Read the model definition and answer for the solid it produces. Units are mm, in the model's axes. A direction names the side the tool comes from. Round coordinates to 2 decimals unless told otherwise and drop trailing zeros. Order: outer loops, then holes, each group sorted by start corner. A loop starts at its lowest first (then second) coordinate and runs counter-clockwise, first axis right, second up. Notation, with made-up numbers: (56, 22) - (75, 22) arc R29 ccw to (75, 47) - close; hole circle Ø9 at (-6, -26.75). An arc over 180 degrees is marked (long way). Put each result on its own line as item: value. Start each with the question number.
Q1. Section B-B on x = 6 is taken. Give the vertices of the cut face in (y, z).
Q2. Section D-D on z = 76 is taken. Give the vertices of the cut face in (x, y).
Q3. For a pull along X with two mould halves and no side action, classify faces 4 (the face through (0, 92, 44)), 5 (the face through (5.916, 125.28, 64.946)), 6 (the face through (6, 75, 67)) as pulls with the +X half, pulls with the -X half, needs draft (parallel to the pull), parting line crosses it, or undercut.
Q4. Find the intervals of material crossed by line 1 along X through (y, z) = (75, 13); line 2 along Y through (x, z) = (4.5, 78); line 3 along Y through (x, z) = (8.5, 11.5), in increasing order. Write a range as from..to.
Q5. Section C-C on z = 22 is taken. Give the vertices of the cut face in (x, y).
Q6. Section A-A on y = 75 is taken. Give the vertices of the cut face in (x, z), then the cut area to 3 significant figures.
Q7. Each of these flat-tipped pins is pushed along its axis until it touches: pin 1 Ø5 at (x, y) = (6, 75) entering from -Z; pin 2 Ø6 at (x, y) = (6.5, 111) entering from +Z; pin 3 Ø5.5 at (x, y) = (6, 75) entering from +Z. Where does it stop, or does it pass through?
Q8. Which of the six approach directions +Z, -Z, +X, -X, +Y, -Y give full straight-line access (tool end or side, diameter ignored) to faces 1 (the face through (5.35, 72.07, 77.14)), 2 (the face through (5.35, 77.93, 12.32)), 3 (the face through (6, 82, 0))?
from build123d import *

# Parameters (mm, degrees)
F1_DEPTH = 12
F2_R     = 3
F3_DEPTH = 20
F4_R     = 3
F5_DEPTH = 25
F6_R     = 2
F7_DEPTH = 25
F8_W     = 60
F8_H     = 87
F9_DEPTH = 25


with BuildPart() as f1:
    # F0 (on Right) → F1 (new body)
    with BuildSketch(Plane.YZ):
        Polygon((0, 87), (0, 0), (105, 0), (145, 43.5), (105, 87), align=None)
    extrude(amount=F1_DEPTH)

    # F2 (on face) → F3 (cut)
    with BuildSketch(Plane.XY.offset(87)):
        with Locations((6, 15)):
            Circle(F2_R)
        with Locations((6, 45)):
            Circle(F2_R)
        with Locations((6, 75)):
            Circle(F2_R)
    extrude(amount=-F3_DEPTH, mode=Mode.SUBTRACT)

    # F4 (on face) → F5 (cut)
    with BuildSketch(Plane(origin=(0, 0, 0), x_dir=(1, 0, 0), z_dir=(0, 0, -1))):
        with BuildLine():
            Line((6, -15), (9, -15))
            ThreePointArc((9, -15), (8.12132, -12.87868), (6, -12))
            Line((6, -12), (6, -15))
        make_face()
        with BuildLine():
            ThreePointArc((9, -45), (8.12132, -42.87868), (6, -42))
            ThreePointArc((6, -42), (3.87868, -47.12132), (9, -45))
        make_face()
        with BuildLine():
            ThreePointArc((6, -18), (8.12132, -17.12132), (9, -15))
            Line((9, -15), (6, -15))
            Line((6, -15), (6, -18))
        make_face()
        with BuildLine():
            Line((6, -15), (6, -12))
            ThreePointArc((6, -12), (3, -15), (6, -18))
            Line((6, -18), (6, -15))
        make_face()
        with Locations((6, -75)):
            Circle(F4_R)
    extrude(amount=-F5_DEPTH, mode=Mode.SUBTRACT)

    # F6 (on face) → F7 (cut)
    with BuildSketch(Plane(origin=(0, 0, 0), x_dir=(0, -1, 0), z_dir=(-1, 0, 0))):
        with Locations((-6, 77)):
            Circle(F6_R)
        with Locations((-6, 10)):
            Circle(F6_R)
    extrude(amount=-F7_DEPTH, mode=Mode.SUBTRACT)

    # F8 (on face) → F9 (cut)
    with BuildSketch(Plane.YZ.offset(12)):
        with Locations((30, 43.5)):
            Rectangle(F8_W, F8_H)
    extrude(amount=-F9_DEPTH, mode=Mode.SUBTRACT)


solid = f1.part
Findings:
1. outline: (60, 0) - (72, 0) - (72, 25) - (78, 25) - (78, 0) - (105, 0) - (145, 43.5) - (105, 87) - (78, 87) - (78, 67) - (72, 67) - (72, 87) - (60, 87) - close
2. outline: (0, 60) - (12, 60) - (12, 115.11) - (0, 115.11) - close; hole circle Ø6 at (6, 75)
3. face 4: pulls with the -X half
3. face 5: needs draft
3. face 6: undercut
4. line 1: 0..3, 9..12
4. line 2: 60..72.4, 77.6..113.28
4. line 3: 60..73.34, 76.66..115.57
5. outline: (0, 60) - (12, 60) - (12, 125.23) - (0, 125.23) - close; hole circle Ø6 at (6, 75)
6. outline: (0, 0) - (3, 0) - (3, 25) - (9, 25) - (9, 0) - (12, 0) - (12, 87) - (9, 87) - (9, 67) - (3, 67) - (3, 87) - (0, 87) - close
6. area: 774 mm2
7. pin 1: z = 25
7. pin 2: z = 83.74
7. pin 3: z = 67
8. face 1: +Z
8. face 2: -Z
8. face 3: -Z, +X, -X, +Y, -Y
